```python
from build123d import *

# Parameters (mm, degrees)
SKETCH1_W              = 5.5
SKETCH1_H              = 2.8
BOSS_EXTRUDE1_DEPTH    = 40
M2_5_CLEARANCE_HOLE1_D = 2.9


with BuildPart() as part:
    # Sketch1 → Boss-Extrude1 (new body)
    with BuildSketch(Plane(origin=(0, 0, 0), x_dir=(1, 0, 0), z_dir=(0, 1, 0))):
        Rectangle(SKETCH1_W, SKETCH1_H)
    extrude(amount=BOSS_EXTRUDE1_DEPTH)

    # M2.5 Clearance Hole1 (through all)
    with Locations(Plane.XY.offset(1.4)):
        with Locations((0, 20), (0, 37), (0, 3)):
            Hole(M2_5_CLEARANCE_HOLE1_D / 2)


solid = part.part
```
Source: CAD feature listing. Evaluate the final solid. Frame: model axes, mm. Give positions to 0.01 mm unless a question says otherwise; leave off trailing zeros. Loops run counter-clockwise (first coordinate to the right, second up) from the corner with the lowest first, then second, coordinate; pieces in that order, holes last. Notation, with made-up numbers: (35, 47) -> (81, 47) arc R20 cw to (81, 54) -> close; hole circle Ø1 at (41, 0.25). An arc over 180 degrees is marked (long way). Put each result on its own line as item: value. Start each with the question number.
1) Cut plane C-C (z = -0.05). Return loops of the section in (x, y), then the cut area to 3 significant figures.
2) Draft query along Y for faces 1 (the face through (-0.669, 35.714, -0.02)), 2 (the face through (-2, 20, -1.4)), 3 (the face through (0, 40, 0)). Return one class per face: released by +Y, released by -Y, zero draft, split by the parting line, or undercut.
3) Material intervals for probe 1 along Y at (x, z) = (0, -0.65); probe 2 along Y at (x, z) = (1.15, 1); probe 3 along X at (y, z) = (21, 1.05), sorted ascending.
4) Cut plane A-A (y = 37). Return loops of the section in (x, z).
5) Cut plane B-B (x = 0). Return loops of the section in (y, z), then the cut area to 3 significant figures.
Results are:
1. outline: (-2.75, 0) -> (2.75, 0) -> (2.75, 40) -> (-2.75, 40) -> close; hole circle Ø2.9 at (0, 3); hole circle Ø2.9 at (0, 20); hole circle Ø2.9 at (0, 37)
1. area: 200 mm2
2. face 1: undercut
2. face 2: zero draft
2. face 3: released by +Y
3. probe 1: y = 0 to 1.55, 4.45 to 18.55, 21.45 to 35.55, 38.45 to 40
3. probe 2: y = 0 to 2.12, 3.88 to 19.12, 20.88 to 36.12, 37.88 to 40
3. probe 3: x = -2.75 to -1.05, 1.05 to 2.75
4. outline: (-2.75, -1.4) -> (-1.45, -1.4) -> (-1.45, 1.4) -> (-2.75, 1.4) -> close; (1.45, -1.4) -> (2.75, -1.4) -> (2.75, 1.4) -> (1.45, 1.4) -> close
5. outline: (0, -1.4) -> (1.55, -1.4) -> (1.55, 1.4) -> (0, 1.4) -> close; (4.45, -1.4) -> (18.55, -1.4) -> (18.55, 1.4) -> (4.45, 1.4) -> close; (21.45, -1.4) -> (35.55, -1.4) -> (35.55, 1.4) -> (21.45, 1.4) -> close; (38.45, -1.4) -> (40, -1.4) -> (40, 1.4) -> (38.45, 1.4) -> close
5. area: 87.6 mm2
